Input: part model. Units: mm. Frame: model coordinates. Face numbers are marked on the shaded views. A direction names the side the tool comes from. Give positions to 0.01 mm unless a question says otherwise; leave off trailing zeros. Loops run counter-clockwise (first coordinate to the right, second up) from the corner with the lowest first, then second, coordinate; pieces in that order, holes last. Notation, with made-up numbers: M -23,17 L 31,17 A18 ccw 31,29 Z; hole C 84.5,60.25 d4. An arc over 180 degrees is marked long. One line per item, written item: value. Start each with the question number.
(1) Section B-B on x = -7. Output: boundary loops of the cut face in (y, z).
(2) Section A-A on z = -3. Output: boundary loops of the cut face in (x, y).
(3) Section C-C on y = 24. Output: boundary loops of the cut face in (x, z).
(4) Ray query, line 1 along X through (y, z) = (15.5, -3); line 2 along Y through (x, z) = (-0.5, 0.5); line 3 along Z through (x, y) = (-6.25, 2.75). Return the intervals inside material, ascending. Write a range as from..to.
(5) Pull-direction query (X, two-part tool) for the marked faces 5, 6, 7 and 8; classes: released by +X, released by -X, zero draft, split by the parting line, or undercut.
(6) Access query for the marked faces 1, 2, 3 and 4. Directions: +Z, -Z, +X, -X, +Y, -Y. A direction counts if a zero-diameter tool reaches every point of the face in a straight line with its end or side. Return the directions, or none.
(7) Pin query (flat end, axial travel): P1, Ø1.5, axis at y = 6, z = 1, coming from the +X side; P2, Ø1.6, axis at x = 3, z = 1, coming from the +Y side; P3, Ø1.5, axis at y = 21, z = -3.5, coming from the -X side; P4, Ø1.1, axis at x = -1, z = 1, coming from the -Y side. Return the tip coordinate at first contact, or that it passes through.
```python
from build123d import *

# Parameters (mm, degrees)
BOSS_SWITCH_BODY_DEPTH            = 3
SKETCH1_W                         = 2.994375291
SKETCH1_H                         = 2.409101515
SKETCH1_W_2                       = 3.994375291
SKETCH1_H_2                       = 3.957767538
BOSS_FLANGE_WIDTH_DEPTH           = 5
BOSS_FLANGE_HEIGHT_REACH          = 36.354
SKETCH2_W                         = 4
SKETCH2_H                         = 3.957767538
SKETCH2_W_2                       = 8
SKETCH2_H_2                       = 1.451333978
SKETCH17_W                        = 15.1675
SKETCH17_H                        = 4
BOSS_FLANGE_SUPPORT_DEPTH         = 13.053634428
CUT_WALL_GAP_DEPTH                = 1
TAP_DRILL_FOR_M2X0_4_TAP1_D       = 1.6
M2_CLEARANCE_HOLE2_D              = 2.4
M2_CLEARANCE_HOLE2_DEPTH          = 13.462735941
CHAMFER_FLANGE_SUPPORT_3_SIZE     = 1
FILLET1_R                         = 1
FILLET2_R                         = 0.5
SKETCH28_W                        = 5.9675
SKETCH28_H                        = 12.095866891
CUT_PRINT_SUPPORT_CLEARANCE_DEPTH = 33.624103931


with BuildPart() as part:
    # Sketch-SwitchBossUp → Boss-Switch Body (new body)
    with BuildSketch(Plane.XY):
        with BuildLine():
            Line((-5.697895702, 26.949658376), (-5.524247524, 25.964850623))
            ThreePointArc((-5.524247524, 25.964850623), (-6.169751391, 25.553619307), (-6.3354071, 24.806394693))
            Line((-6.3354071, 24.806394693), (-4.07798079, 12.003893904))
            ThreePointArc((-4.07798079, 12.003893904), (-3.666749473, 11.358390037), (-2.919524859, 11.192734328))
            Line((-2.919524859, 11.192734328), (-2.755222696, 10.260930457))
            Line((-2.755222696, 10.260930457), (-1.920417042, 9.937339624))
            Line((-1.920417042, 9.937339624), (-1.291045382, 9.693379968))
            Line((-1.291045382, 9.693379968), (-1.735258621, 8.547390389))
            ThreePointArc((-1.735258621, 8.547390389), (-1.752158006, 8.457034961), (-1.735258621, 8.366679532))
            Line((-1.735258621, 8.366679532), (-1.291045382, 7.220689953))
            Line((-1.291045382, 7.220689953), (-1.920417042, 6.976730297))
            Line((-1.920417042, 6.976730297), (-0.547014535, 3.433600952))
            Line((-0.547014535, 3.433600952), (0.082357125, 3.677560608))
            Line((0.082357125, 3.677560608), (0.805200549, 1.81275569))
            Line((0.805200549, 1.81275569), (-0.12720191, 1.451333978))
            Line((-0.12720191, 1.451333978), (-0.12720191, 0))
            Line((-0.12720191, 0), (2.867173381, 0))
            Line((2.867173381, 0), (2.867173381, 2.409101515))
            Line((2.867173381, 2.409101515), (2.343664607, 2.409101515))
            Line((2.343664607, 2.409101515), (1.411262148, 2.047679803))
            Line((1.411262148, 2.047679803), (0.688418723, 3.912484721))
            Line((0.688418723, 3.912484721), (1.317790383, 4.156444377))
            Line((1.317790383, 4.156444377), (1.081123773, 4.767001302))
            Line((1.081123773, 4.767001302), (3.143260738, 5.566335394))
            Line((3.143260738, 5.566335394), (3.143260738, 6.901787438))
            Line((3.143260738, 6.901787438), (2.24307649, 7.888306327))
            Line((2.24307649, 7.888306327), (0.181054486, 7.089016797))
            Line((0.181054486, 7.089016797), (-0.055612124, 7.699573722))
            Line((-0.055612124, 7.699573722), (-0.684983784, 7.455614066))
            Line((-0.684983784, 7.455614066), (-1.038134762, 8.366679532))
            ThreePointArc((-1.038134762, 8.366679532), (-1.055034148, 8.457034961), (-1.038134762, 8.547390389))
            Line((-1.038134762, 8.547390389), (-0.684983784, 9.458455855))
            Line((-0.684983784, 9.458455855), (-0.055612124, 9.214496199))
            Line((-0.055612124, 9.214496199), (1.317790383, 12.757625544))
            Line((1.317790383, 12.757625544), (0.688418723, 13.0015852))
            Line((0.688418723, 13.0015852), (1.411262148, 14.866390118))
            Line((1.411262148, 14.866390118), (2.343664607, 14.504968406))
            Line((2.343664607, 14.504968406), (2.867173381, 14.504968406))
            Line((2.867173381, 14.504968406), (2.867173381, 18.462735944))
            Line((2.867173381, 18.462735944), (-0.111637615, 18.462735944))
            Line((-0.111637615, 18.462735944), (-1.12720191, 18.462735944))
            Line((-1.12720191, 18.462735944), (-1.12720191, 15.462735944))
            Line((-1.12720191, 15.462735944), (-0.12720191, 15.462735944))
            Line((-0.12720191, 15.462735944), (0.805200549, 15.101314231))
            Line((0.805200549, 15.101314231), (0.082357125, 13.236509313))
            Line((0.082357125, 13.236509313), (-0.547014535, 13.480468969))
            Line((-0.547014535, 13.480468969), (-1.059112089, 12.159350171))
            Line((-1.059112089, 12.159350171), (-2.346896051, 19.462735944))
            Line((-2.346896051, 19.462735944), (3.767173381, 19.462735944))
            Line((3.767173381, 19.462735944), (3.767173381, 25.857619356))
            Line((3.767173381, 25.857619356), (1.767173381, 25.857619356))
            Line((1.767173381, 25.857619356), (1.767173381, 21.462735944))
            Line((1.767173381, 21.462735944), (-2.699550012, 21.462735944))
            Line((-2.699550012, 21.462735944), (-3.728280196, 27.296954732))
            ThreePointArc((-3.728280196, 27.296954732), (-2.874356585, 27.992742953), (-2.319025652, 28.944012807))
            ThreePointArc((-2.319025652, 28.944012807), (-2.76728001, 29.905297381), (-3.728564583, 29.457043022))
            ThreePointArc((-3.728564583, 29.457043022), (-4.944660137, 28.436617692), (-6.436422172, 28.97957467))
            ThreePointArc((-6.436422172, 28.97957467), (-7.493046212, 29.072017295), (-7.585488837, 28.015393255))
            ThreePointArc((-7.585488837, 28.015393255), (-6.738295005, 27.311426358), (-5.697895702, 26.949658376))
        make_face()
    extrude(amount=BOSS_SWITCH_BODY_DEPTH)

    # Sketch1 → Boss-Flange Width (add)
    with BuildSketch(Plane(origin=(0, 0, 0), x_dir=(-1, 0, 0), z_dir=(0, 0, -1))):
        with Locations((-1.369985736, 1.204550758)):
            Rectangle(SKETCH1_W, SKETCH1_H)
        with Locations((-0.869985736, 16.483852175)):
            Rectangle(SKETCH1_W_2, SKETCH1_H_2)
    extrude(amount=BOSS_FLANGE_WIDTH_DEPTH)

    # Boss-Flange Height: up to this face of the body (flat: up to its plane)
    boss_flange_height_end = Plane(part.part.faces().sort_by_distance((-0.12720191, 1.077409098, -1.438016547))[0])
    # Sketch2 → Boss-Flange Height (add, up to the picked face)
    with BuildSketch(Plane(origin=(-12.300326619, 0, 0), x_dir=(0, 0, -1), z_dir=(1, 0, 0)), mode=Mode.PRIVATE) as boss_flange_height_sk1:
        with Locations((3, 16.483852175)):
            Rectangle(SKETCH2_W, SKETCH2_H)
    boss_flange_height_tool1 = split(extrude(boss_flange_height_sk1.sketch, amount=BOSS_FLANGE_HEIGHT_REACH, mode=Mode.PRIVATE), bisect_by=boss_flange_height_end, keep=Keep.BOTH, mode=Mode.PRIVATE)
    # Sketch2 → Boss-Flange Height (add, up to the picked face)
    with BuildSketch(Plane(origin=(-12.300326619, 0, 0), x_dir=(0, 0, -1), z_dir=(1, 0, 0)), mode=Mode.PRIVATE) as boss_flange_height_sk2:
        with Locations((1, 0.725666989)):
            Rectangle(SKETCH2_W_2, SKETCH2_H_2)
    boss_flange_height_tool2 = split(extrude(boss_flange_height_sk2.sketch, amount=BOSS_FLANGE_HEIGHT_REACH, mode=Mode.PRIVATE), bisect_by=boss_flange_height_end, keep=Keep.BOTH, mode=Mode.PRIVATE)
    add(boss_flange_height_tool1.solids().sort_by(Axis((-12.300327, 16.483852, -3), (1, 0, 0)))[0])
    add(boss_flange_height_tool2.solids().sort_by(Axis((-12.300327, 0.725667, -1), (1, 0, 0)))[0])

    # Sketch17 → Boss-Flange Support (add)
    with BuildSketch(Plane.XZ.offset(-1.451333978)):
        with Locations((-4.716576619, -3)):
            Rectangle(SKETCH17_W, SKETCH17_H)
    extrude(amount=-BOSS_FLANGE_SUPPORT_DEPTH)

    # Sketch27 → Cut-Wall Gap (cut)
    with BuildSketch(Plane.XY):
        Polygon((-0.12720191, 15.462735944), (2.343664607, 14.504968406), (-1.12720191, 14.504968406), (-1.12720191, 15.462735944), align=None)
        Polygon((2.343664607, 2.409101515), (-0.12720191, 2.409101515), (-0.12720191, 1.451333978), align=None)
    extrude(amount=-CUT_WALL_GAP_DEPTH, mode=Mode.SUBTRACT)

    # Tap Drill for M2x0.4 Tap1 (through all)
    with Locations(Plane(origin=(0, 0, 0), x_dir=(-1, 0, 0), z_dir=(0, -1, 0))):
        with Locations((9.300326619, 3), (5.300326619, 3)):
            Hole(TAP_DRILL_FOR_M2X0_4_TAP1_D / 2)

    # M2 Clearance Hole2
    with Locations(Plane.XZ):
        with Locations((-9.300326619, -3), (-5.300326619, -3)):
            Hole(M2_CLEARANCE_HOLE2_D / 2, depth=M2_CLEARANCE_HOLE2_DEPTH)

    # Chamfer-Flange Support 3
    chamfer_flange_support_3_edges = [part.edges().sort_by_distance(p)[0] for p in [
        (-6.213764264, 1.451333978, -1),
    ]]
    chamfer(chamfer_flange_support_3_edges, length=CHAMFER_FLANGE_SUPPORT_3_SIZE)

    # Fillet1
    fillet1_edges = [part.edges().sort_by_distance(p)[0] for p in [
        (-2.755222696, 10.260930457, 1.5),
    ]]
    fillet(fillet1_edges, radius=FILLET1_R)

    # Fillet2
    fillet2_edges = [part.edges().sort_by_distance(p)[0] for p in [
        (-1.920417042, 6.976730297, 1.5),
    ]]
    fillet(fillet2_edges, radius=FILLET2_R)

    # Sketch28 → Cut-Print Support Clearance (cut, through all)
    with BuildSketch(Plane.XY.offset(-1)):
        with Locations((-0.116576619, 8.457034961)):
            Rectangle(SKETCH28_W, SKETCH28_H)
    extrude(amount=-CUT_PRINT_SUPPORT_CLEARANCE_DEPTH, mode=Mode.SUBTRACT)


solid = part.part
```
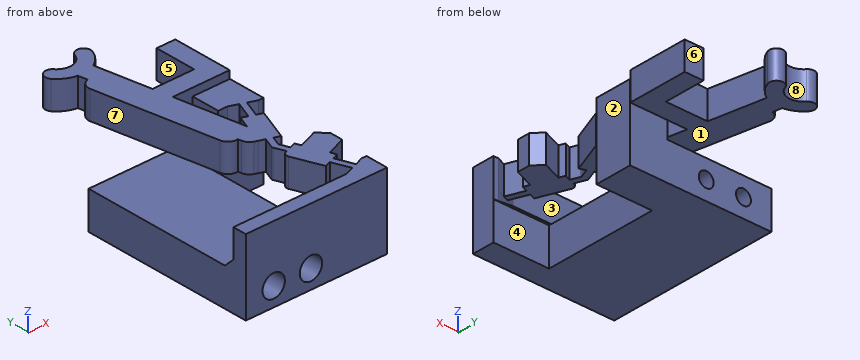
Output values:
1. outline: M 0,-5 L 18.46,-5 L 18.46,-1 L 2.45,-1 L 1.45,0 L 1.45,3 L 0,3 Z; M 27.48,0 L 29.25,0 L 29.25,3 L 27.48,3 Z
2. outline: M -12.3,0 L -10.5,0 L -10.5,13.46 L -10.1,13.46 L -10.1,18.46 L -12.3,18.46 Z; M -8.5,13.46 L -8.1,13.46 L -8.1,0 L -6.5,0 L -6.5,13.46 L -6.1,13.46 L -6.1,18.46 L -8.5,18.46 Z; M -4.5,13.46 L -4.1,13.46 L -4.1,0 L 2.87,0 L 2.87,2.41 L -3.1,2.41 L -3.1,14.5 L 2.87,14.5 L 2.87,18.46 L -4.5,18.46 Z
3. outline: M -6.19,0 L -3.15,0 L -3.15,3 L -6.19,3 Z; M 1.77,0 L 3.77,0 L 3.77,3 L 1.77,3 Z
4. line 1: x = -12.3..-10.1, -8.5..-6.1, -4.5..2.87
4. line 2: y = 0..1.45, 3.45..7.53, 9.39..13.46, 15.46..18.46, 19.46..21.46
4. line 3: z = -5..-3.73, -2.27..-1
5. face 5: undercut
5. face 6: zero draft
5. face 7: released by -X
5. face 8: undercut
6. face 1: -X
6. face 2: +Z, -Z, +X
6. face 3: +Z, -X
6. face 4: -Z, +X
7. P1: stops at x = 3.14
7. P2: stops at y = 25.86
7. P3: passes through
7. P4: stops at y = 0
